Design review of the part shown in the three views and the two pictorial views. Dimensions are in mm from the part's minimum x, y and z. Coordinates: 2 decimals unless noted, no trailing zeros. Order: outer loops, then holes, each group sorted by start corner. A loop starts at its lowest first (then second) coordinate and runs counter-clockwise, first axis right, second up. Notation, with made-up numbers: (26.5, 33.25) -> (58.5, 33.25) arc R11 cw to (58.5, 54.25) -> close; hole circle Ø6 at (27.25, 60). An arc over 180 degrees is marked (long way). Answer as a JSON object with one key per item and string values. Group by question number.
1) Wall thickness on L1, parallel to Y at x = 31, z = 29 (1 decimal); L2, parallel to Z at x = 10.5, y = 51; L3, parallel to X at y = 45, z = 13: over which ranges is each line inside the solid? List them lowest first.
2) For pin 1 (10 mm diameter, centred on y = 39.5, z = 17, fed in from -X); pin 2 (1 mm diameter, centred on x = 23.5, z = 15.5, fed in from +Y); pin 3 (1 mm diameter, centred on x = 54, y = 25.5, fed in from -Z); pin 4 (5 mm diameter, centred on x = 32.5, y = 41.5, fed in from -Z), all flat-tipped, find the tip position at first contact; note any pin that passes through.
3) Add section A-A, the plane y = 34. Write out the cut boundary in (x, z).
4) Draft analysis for pull direction Y (two halves, no side actions). For the marked faces 1, 2 and 3, state which applies: +Y half, -Y half, draft (parallel to the pull), parting line (faces both ways), or undercut.
5) Add section C-C, the plane z = 13. Write out the cut boundary in (x, y), then the cut area to 3 significant figures.
6) Add section D-D, the plane x = 7.5. Write out the cut boundary in (y, z).
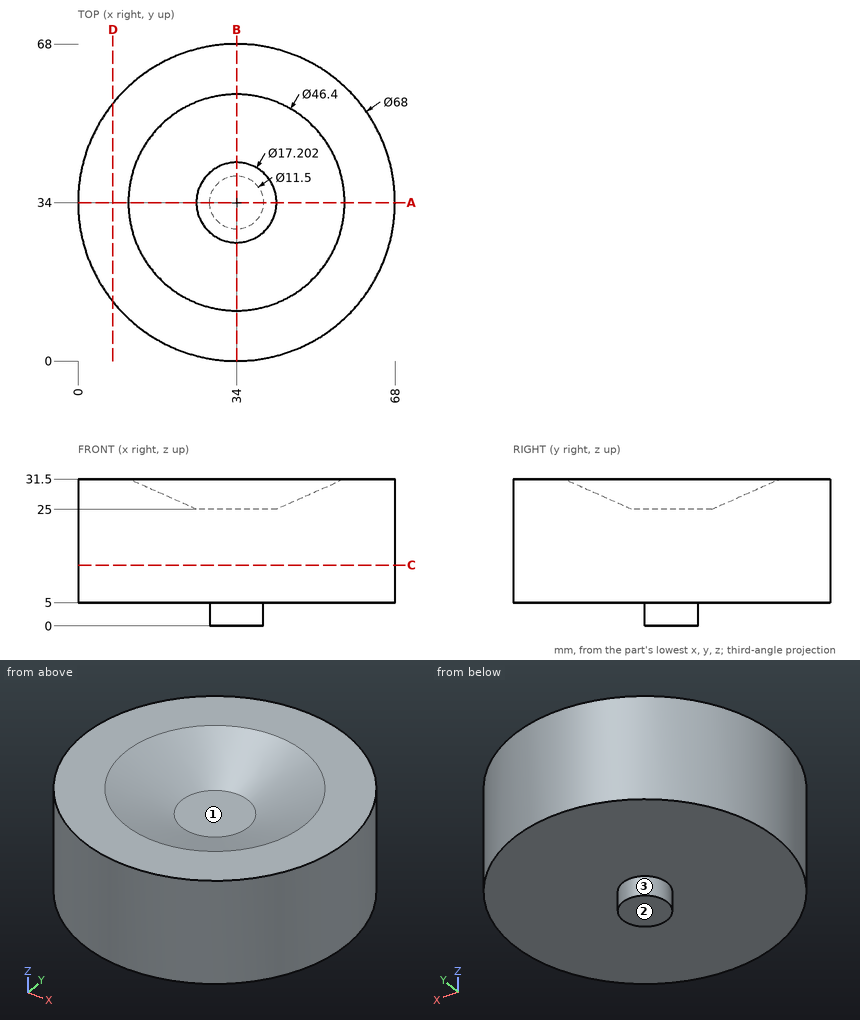
Output values:
{
 "1": {"L1": "y = 0.1 to 16.7, 51.3 to 67.9", "L2": "z = 5 to 31.5", "L3": "x = 1.83 to 66.17"},
 "2": {"pin 1": "stops at x = 0", "pin 2": "stops at y = 66.5", "pin 3": "stops at z = 5", "pin 4": "stops at z = 0"},
 "3": {"outline": "(0, 5) -> (28.25, 5) -> (28.25, 0) -> (39.75, 0) -> (39.75, 5) -> (68, 5) -> (68, 31.5) -> (57.2, 31.5) -> (42.6, 25) -> (25.4, 25) -> (10.8, 31.5) -> (0, 31.5) -> close"},
 "4": {"face 1": "undercut", "face 2": "draft", "face 3": "parting line"},
 "5": {"outline": "circle Ø68 at (34, 34)", "area": "3,630 mm²"},
 "6": {"outline": "(12.7, 5) -> (55.3, 5) -> (55.3, 31.5) -> (12.7, 31.5) -> close"}
}
